Here's how the part is built. I have some questions about the finished solid (model axes, mm). Coordinates: 2 decimals unless noted, no trailing zeros. Loops run counter-clockwise (first coordinate to the right, second up) from the corner with the lowest first, then second, coordinate; pieces in that order, holes last. Notation, with made-up numbers: (23, 43) -> (72, 43) arc R19 ccw to (72, 53) -> close; hole circle Ø9 at (-12, -14). An arc over 180 degrees is marked (long way). Answer as a JSON object with one key per item and string values. Group by question number.
1) I need wall thicknesses on probe 1 along X at (y, z) = (15, 11.5); probe 2 along X at (y, z) = (17, 6). Which ranges of each line are inside material? Lowest first, please. Write a range as [from, to].
2) I'm going to push a flat-ended pin straight in: pin 1 (8 mm diameter, centred on y = 7.5, z = 13, fed in from -X). Where does the tip first touch, or does it pass through?
3) I want a section at C-C (z = 5.75). Write out the boundary of the cut face in (x, y).
4) I want a section at A-A (x = 15). Write out the boundary of the cut face in (y, z).
5) If we mould it in two halves opening along X, with no side actions, what happens to faces 1 (the flat face through (15, 30, 7)), 2 (the cylindrical face through (11.767, 16.341, 7.605)), 3 (the flat face through (30, 15, 7))? For each: +X half, -X half, draft (parallel to the pull), parting line (faces both ways), or undercut.
Autodesk Fusion 360 part; units mm, degrees
sketch "Skizze1" plane through (0, 0, 0) normal (0, 0, 1) x (1, 0, 0)
  line L0 (0, 0) -> (30, 0)
  line L1 (30, 0) -> (30, 30)
  line L2 (30, 30) -> (0, 30)
  line L3 (0, 30) -> (0, 0)
  dimension "d1" = 30
  dimension "d2" = 30
extrude "Extrusion1" add sketch "Skizze1" along normal blind 15
sketch "Skizze2" plane through (0, 0, 15) normal (0, 0, 1) x (-1, 0, 0)
  line L0 (0, -30) -> (0, 0)
  line L1 (0, 0) -> (-30, 0)
  line L2 (-30, 0) -> (-30, -30)
  line L3 (-30, -30) -> (0, -30)
  circle A0 centre (-15, -15) radius 3.5
  dimension "d5" = 7
extrude "Extrusion2" cut sketch "Skizze2" against normal blind 15 contours A0
Determined:
{
 "1": {"probe 1": "[0, 11.5], [18.5, 30]", "probe 2": "[0, 12.13], [17.87, 30]"},
 "2": {"pin 1": "x = 0"},
 "3": {"outline": "(0, 0) -> (30, 0) -> (30, 30) -> (0, 30) -> close; hole circle Ø7 at (15, 15)"},
 "4": {"outline": "(0, 0) -> (11.5, 0) -> (11.5, 15) -> (0, 15) -> close; (18.5, 0) -> (30, 0) -> (30, 15) -> (18.5, 15) -> close"},
 "5": {"face 1": "draft", "face 2": "undercut", "face 3": "+X half"}
}
